from build123d import *

# Parameters (mm, degrees)
SKETCH1_W           = 90
SKETCH1_H           = 70
BOSS_EXTRUDE1_DEPTH = 60
SKETCH2_W           = 60
SKETCH2_H           = 40
CUT_EXTRUDE1_DEPTH  = 40
SKETCH3_W           = 30
SKETCH3_H           = 30
CUT_EXTRUDE2_DEPTH  = 10
SKETCH4_W           = 30
SKETCH4_H           = 10
CUT_EXTRUDE3_DEPTH  = 20
SKETCH5_W           = 10
SKETCH5_H           = 20
CUT_EXTRUDE4_DEPTH  = 10
SKETCH7_W           = 40
SKETCH7_H           = 30
CUT_EXTRUDE5_DEPTH  = 20
CHAMFER1_SIZE       = 20


with BuildPart() as part:
    # Sketch1 → Boss-Extrude1 (new body)
    with BuildSketch(Plane(origin=(0, 0, 0), x_dir=(1, 0, 0), z_dir=(0, 1, 0))):
        with Locations((45, 35)):
            Rectangle(SKETCH1_W, SKETCH1_H)
    extrude(amount=BOSS_EXTRUDE1_DEPTH)

    # Sketch2 → Cut-Extrude1 (cut)
    with BuildSketch(Plane(origin=(0, 60, 0), x_dir=(1, 0, 0), z_dir=(0, 1, 0))):
        with Locations((30, 20)):
            Rectangle(SKETCH2_W, SKETCH2_H)
    extrude(amount=-CUT_EXTRUDE1_DEPTH, mode=Mode.SUBTRACT)

    # Sketch3 → Cut-Extrude2 (cut)
    with BuildSketch(Plane(origin=(0, 20, 0), x_dir=(1, 0, 0), z_dir=(0, 1, 0))):
        with Locations((15, 15)):
            Rectangle(SKETCH3_W, SKETCH3_H)
    extrude(amount=-CUT_EXTRUDE2_DEPTH, mode=Mode.SUBTRACT)

    # Sketch4 → Cut-Extrude3 (cut)
    with BuildSketch(Plane.ZY):
        with Locations((-15, 5)):
            Rectangle(SKETCH4_W, SKETCH4_H)
    extrude(amount=-CUT_EXTRUDE3_DEPTH, mode=Mode.SUBTRACT)

    # Sketch5 → Cut-Extrude4 (cut)
    with BuildSketch(Plane.ZY):
        with Locations((-35, 10)):
            Rectangle(SKETCH5_W, SKETCH5_H)
    extrude(amount=-CUT_EXTRUDE4_DEPTH, mode=Mode.SUBTRACT)

    # Sketch7 → Cut-Extrude5 (cut)
    with BuildSketch(Plane(origin=(0, 60, 0), x_dir=(1, 0, 0), z_dir=(0, 1, 0))):
        with Locations((20, 55)):
            Rectangle(SKETCH7_W, SKETCH7_H)
    extrude(amount=-CUT_EXTRUDE5_DEPTH, mode=Mode.SUBTRACT)

    # Chamfer1
    chamfer1_edges = [part.edges().sort_by_distance(p)[0] for p in [
        (75, 60, 0),
    ]]
    chamfer(chamfer1_edges, length=CHAMFER1_SIZE)


solid = part.part
Could you check a few things on this model? Use its own coordinates, in mm. A direction names the side the tool comes from. Give positions to 0.01 mm unless a question says otherwise; leave off trailing zeros. Order: outer loops, then holes, each group sorted by start corner. A loop starts at its lowest first (then second) coordinate and runs counter-clockwise, first axis right, second up. Notation, with made-up numbers: (-28.5, -9.5) - (-24.5, -9.5) arc R24 cw to (-24.5, 14.5) - close; hole circle Ø7 at (-21, 59.25). An arc over 180 degrees is marked (long way). Return JSON: item names as keys, results as strings. Group by question number.
Q1. Please list where these lines run through material, in increasing order: line 1 along Z through (x, y) = (43, 23); line 2 along X through (y, z) = (13, -36.5); line 3 along X through (y, z) = (7, -4.5). Write a range as [from, to].
Q2. Will these pins go through, and if not, where does the flat tip stop? pin 1 Ø18 at (x, y) = (35, 30.5) entering from +Z; pin 2 Ø2 at (y, z) = (37, -35) entering from -X; pin 3 Ø11 at (y, z) = (14.5, -34) entering from -X.
Q3. Which directions (+Z, -Z, +X, -X, +Y, -Y) give clear straight access to the entire face, cutting with the end or side of a thin tool? Please do faces 1 (the face through (0, 20, -55)), 2 (the face through (20, 40, -55)), 3 (the face through (60, 40, -20)), 4 (the face through (90, 30, -35)), 5 (the face through (10, 10, -35)).
Q4. Suppose I cut it at A-A, the plane z = -34. Please give me the cut outline in (x, y), and give its area (3 significant figures).
Q5. Suppose I cut it at B-B, the plane y = 5.5. Please give me the cut outline in (x, z).
Q6. Suppose I cut it at D-D, the plane x = 25. Please give me the cut outline in (y, z), and give its area (3 significant figures).
Q7. Suppose I cut it at C-C, the plane x = 84. Please give me the cut outline in (y, z), and give its area (3 significant figures).
Resolved:
{
 "1": {"line 1": "z = [-70, -40]", "line 2": "x = [10, 90]", "line 3": "x = [20, 90]"},
 "2": {"pin 1": "stops at z = -40", "pin 2": "stops at x = 60", "pin 3": "stops at x = 10"},
 "3": {"face 1": "+Z, -Z, -X, +Y, -Y", "face 2": "+Z, -Z, -X, +Y", "face 3": "+Z, -X, +Y", "face 4": "+Z, -Z, +X, +Y, -Y", "face 5": "+Z, -X, +Y, -Y"},
 "4": {"outline": "(10, 0) - (90, 0) - (90, 60) - (60, 60) - (60, 20) - (10, 20) - close", "area": "2,800 mm2"},
 "5": {"outline": "(0, -70) - (90, -70) - (90, 0) - (20, 0) - (20, -30) - (10, -30) - (10, -40) - (0, -40) - close"},
 "6": {"outline": "(0, -70) - (40, -70) - (40, -40) - (20, -40) - (20, -30) - (10, -30) - (10, 0) - (0, 0) - close", "area": "1,700 mm2"},
 "7": {"outline": "(0, -70) - (60, -70) - (60, -20) - (40, 0) - (0, 0) - close", "area": "4,000 mm2"}
}
